Geometry check sheet. Reference: the model listing, model coordinates, mm. Face numbers are marked on the shaded views. A direction names the side the tool comes from. Coordinates: 2 decimals unless noted, no trailing zeros. Loops run counter-clockwise (first coordinate to the right, second up) from the corner with the lowest first, then second, coordinate; pieces in that order, holes last.
from build123d import *

# Parameters (mm, degrees)
F1_DEPTH = 63.5
F2_DEPTH = 25.4
F3_DEPTH = 7.9375
F5_R     = 6.35


with BuildPart() as f1:
    # F0 (on Front) → F1 (new body, symmetric)
    with BuildSketch(Plane.XZ):
        Polygon((-41.275, -9.525), (41.275, -9.525), (41.275, 9.525), (22.225, 9.525), (-41.275, 9.525), align=None)
    extrude(amount=F1_DEPTH, both=True)

    # F0 (on Front) → F2 (join, symmetric)
    with BuildSketch(Plane.XZ):
        with BuildLine():
            Line((22.225, 9.525), (41.275, 9.525))
            Line((41.275, 9.525), (41.275, 27.0002))
            ThreePointArc((41.275, 27.0002), (45.9246798487, 38.2255201513), (57.15, 42.8752))
            Line((57.15, 42.8752), (60.325, 42.8752))
            Line((60.325, 42.8752), (60.325, 61.9252))
            Line((60.325, 61.9252), (57.15, 61.9252))
            add(Edge.make_bspline(
                [(55.950364042, 61.9045908208), (56.3494203194, 61.9119140361), (56.7493016333, 61.9187812014), (57.15, 61.9252)],
                knots=[110.7227393915, 110.7227393915, 110.7227393915, 110.7227393915, 111.5045361635, 111.5045361635, 111.5045361635, 111.5045361635], degree=3))
            ThreePointArc((55.950364042, 61.9045908208), (32.0337412138, 51.2680628969), (22.225, 27.0002))
            Line((22.225, 27.0002), (22.225, 9.525))
        make_face()
    extrude(amount=F2_DEPTH, both=True)

    # F0 (on Front) → F3 (join, symmetric)
    with BuildSketch(Plane.XZ):
        with BuildLine():
            add(Edge.make_bspline(
                [(-41.275, 9.525), (-40.5345981749, 50.6828617224), (-0.5663750684, 60.8674332248), (55.950364042, 61.9045908208)],
                knots=[0, 0, 0, 0, 110.7227393915, 110.7227393915, 110.7227393915, 110.7227393915], degree=3))
            Line((-41.275, 9.525), (22.225, 9.525))
            Line((22.225, 9.525), (22.225, 27.0002))
            ThreePointArc((22.225, 27.0002), (32.0337412138, 51.2680628969), (55.950364042, 61.9045908208))
        make_face()
    extrude(amount=F3_DEPTH, both=True)

    # F0 (on Front) → F4 (revolve)
    with BuildSketch(Plane.XZ):
        Polygon((60.325, 61.9252), (60.325, 42.8752), (85.725, 42.8752), (85.725, 47.9196608067), (85.725, 61.9252), align=None)
    revolve(axis=Axis((60.325, 0, 52.3875), (0, 0, 1)))

    # F5
    f5_edges = [f1.edges().sort_by_distance(p)[0] for p in [
        (41.275, -63.5, 0),
        (-41.275, -63.5, 0),
        (41.275, 63.5, 0),
        (-41.275, 63.5, 0),
    ]]
    fillet(f5_edges, radius=F5_R)


solid = f1.part
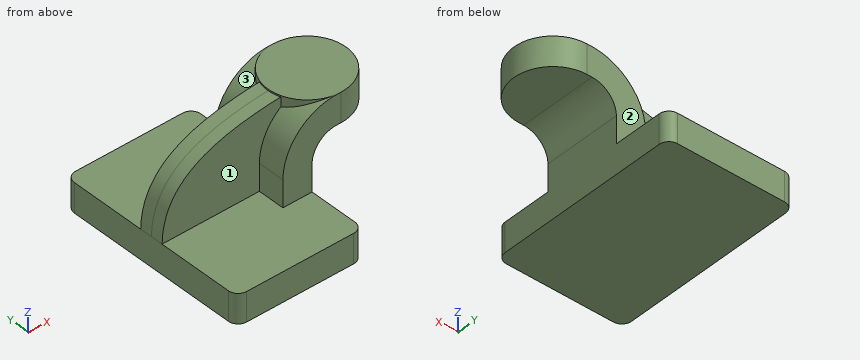
(1) Gauge pin test, flat ends, axial feed: pin 1 Ø14.5 at (x, y) = (66.5, 12.5) entering from -Z; pin 2 Ø5 at (y, z) = (-19.5, 18.5) entering from -X (3 decimals); pin 3 Ø19 at (x, z) = (46, 24) entering from +Y; pin 4 Ø1.5 at (x, z) = (62.5, 42) entering from -Y. Record the tip position at first contact, or that the pin passes through.
Findings:
pin 1: stops at z = 42.88
pin 2: stops at x = 22.225
pin 3: stops at y = 25.4
pin 4: passes through
(2) Sectioned sample at B-B on x = 72. Record the cut outline in (y, z).
Findings:
outline: (-22.56, 42.88) - (22.56, 42.88) - (22.56, 61.93) - (-22.56, 61.93) - close
(3) Access from +Z, -Z, +X, -X, +Y, -Y to the whole of each face (thin tool, end or side, straight path). Record for the marked faces 1, 2 and 3.
Findings:
face 1: +Z, -X, -Y
face 2: +Z, +X, -X, +Y
face 3: +Z, -X, +Y
(4) Scan lines: L1, parallel to Y at x = 16.5, z = 54; L2, parallel to Y at x = 44.5, z = 58; L3, parallel to X at y = -9, z = 1 (3 decimals). Record each from-to range of solid material in increasing order.
Findings:
L1: y = -7.94 to 7.94
L2: y = -25.4 to 25.4
L3: x = -41.275 to 41.275
(5) Sectioned sample at A-A on x = 53. Record the cut outline in (y, z).
Findings:
outline: (-25.4, 42.32) - (25.4, 42.32) - (25.4, 61.68) - (24.32, 61.68) - (24.32, 61.93) - (-24.32, 61.93) - (-24.32, 61.68) - (-25.4, 61.68) - close
